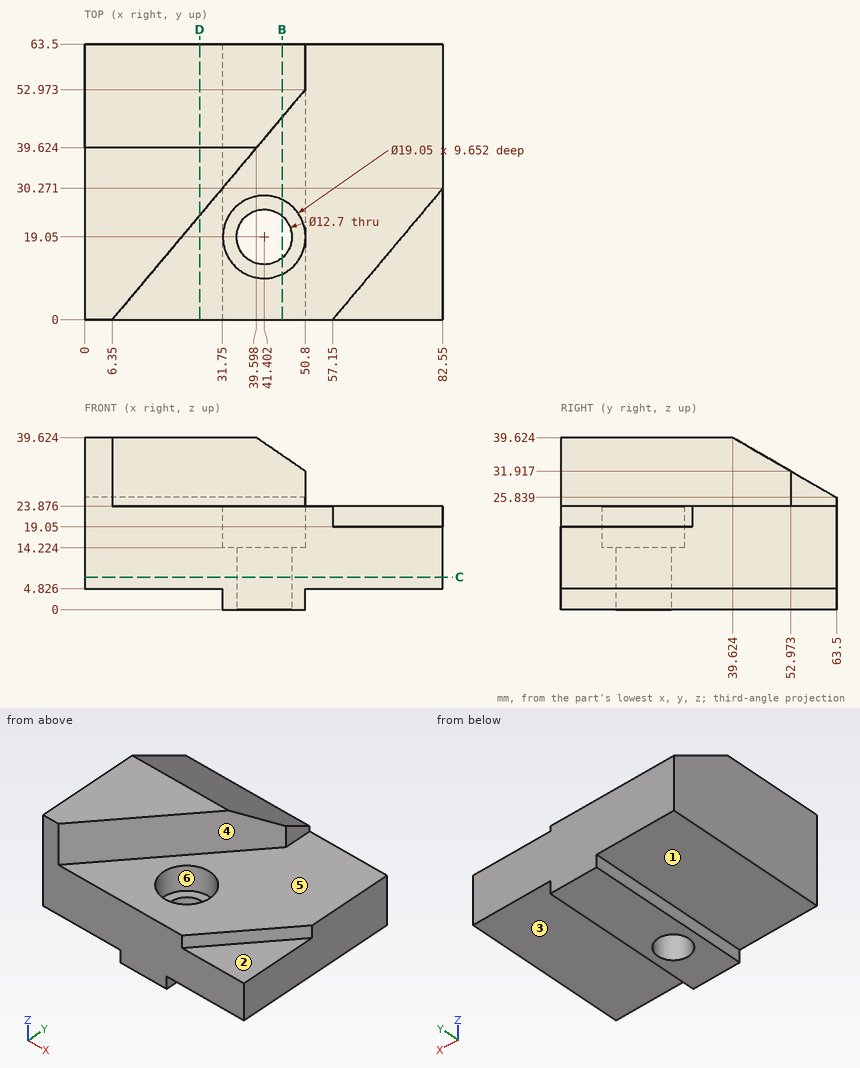
Geometry: see drawing. Coordinates: mm, zero at the bounding-box minimum. A direction names the side the tool comes from. Give positions to 0.01 mm unless a question says otherwise; leave off trailing zeros. Write each loop counter-clockwise with the first axis right and the second up, starting at its lowest first coordinate (ties: lowest second). Pieces come first, ordered by that corner, then holes. Notation, with made-up numbers: M -33.5,11.25 L 25.5,11.25 A27 ccw 25.5,41.25 Z; hole C 12,58.25 d10. An arc over 180 degrees is marked long. Answer as a JSON object with one key per item and string values.
Q1. Cut plane D-D, the plane x = 26.5. Return the cut outline in (y, z), then the cut area to 3 significant figures.
Geometry check:
{"outline": "M 0,4.83 L 63.5,4.83 L 63.5,25.84 L 39.62,39.62 L 24.01,39.62 L 24.01,23.88 L 0,23.88 Z", "area": "1,670 mm^2"}
Q2. Access query for the marked faces 1, 2 and 3. Directions: +Z, -Z, +X, -X, +Y, -Y. A direction counts if a zero-diameter tool reaches every point of the face in a straight line with its end or side. Return the directions, or none.
Geometry check:
{"face 1": "-Z, -X, +Y, -Y", "face 2": "+Z, +X, -Y", "face 3": "-Z, +X, +Y, -Y"}
Q3. Ray query, line 1 along X through (y, z) = (19, 16); line 2 along Z through (x, y) = (25, 18.5); line 3 along Z through (x, y) = (34.5, 32). Return the intervals inside material, ascending.
Geometry check:
{"line 1": "x = 0 to 31.88, 50.93 to 82.55", "line 2": "z = 4.83 to 23.88", "line 3": "z = 0 to 23.88"}
Q4. Mould query, pull axis Y, two halves, no side actions, for the marked faces 4, 5 and 6. Classes: +Y half, -Y half, draft (parallel to the pull), parting line (faces both ways), or undercut.
Geometry check:
{"face 4": "-Y half", "face 5": "draft", "face 6": "undercut"}
Q5. Contact query for flat-ended pins moving along their axis: P1, Ø1, axis at y = 37.5, z = 26.5, coming from the +X side (1 decimal); P2, Ø2, axis at x = 24, y = 55, coming from the +Z side (1 decimal); P3, Ø11.5, axis at x = 41.402, y = 19.05, coming from the -Z side; P4, Ø2.5, axis at y = 39, z = 1.5, coming from the -X side. Output: stop coordinate, or through.
Geometry check:
{"P1": "stops at x = 38.2", "P2": "stops at z = 31.3", "P3": "passes through", "P4": "stops at x = 31.75"}
Q6. Cut plane B-B, the plane x = 45.5. Return the cut outline in (y, z), then the cut area to 3 significant figures.
Geometry check:
{"outline": "M 0,0 L 14.2,0 L 14.2,14.22 L 10.45,14.22 L 10.45,23.88 L 0,23.88 Z; M 23.9,0 L 63.5,0 L 63.5,25.84 L 46.66,35.56 L 46.66,23.88 L 27.65,23.88 L 27.65,14.22 L 23.9,14.22 Z", "area": "1,330 mm^2"}
Q7. Cut plane C-C, the plane z = 7.5. Return the cut outline in (x, y).
Geometry check:
{"outline": "M 0,0 L 82.55,0 L 82.55,63.5 L 0,63.5 Z; hole C 41.4,19.05 d12.7"}
